from build123d import *

# Parameters (mm, degrees)
SM_BASE_FLANGE_2_DEPTH        = 349
CUT_EXTRUDE_1_DEPTH           = 10
PATTERN_LINEAR_1_COUNT        = 2
PATTERN_LINEAR_1_PITCH        = 251
PATTERN_LINEAR_1_COPY_1_DEPTH = 10


# Sheet-metal steps are written as plain solids
with BuildPart() as part:
    # 草图2 → 基体-法兰2 (new body)
    with BuildSketch(Plane(origin=(0, 0, 0), x_dir=(0, 0, -1), z_dir=(1, 0, 0))):
        Polygon((0, 0), (0, 45.845517328), (4.75, 54.072758664), (5.702627944, 53.522758664), (1.1, 45.550773216), (1.1, 0.294744112), (5.702627944, -7.677241336), (4.75, -8.227241336), align=None)
    extrude(amount=-SM_BASE_FLANGE_2_DEPTH)

    # 草图11 → 切除-拉伸1 (cut)
    with BuildSketch(Plane.XY):
        with BuildLine():
            Line((-46, 14.922758664), (-46, 10.922758664))
            ThreePointArc((-46, 10.922758664), (-49, 7.922758664), (-52, 10.922758664))
            Line((-52, 10.922758664), (-52, 14.922758664))
            ThreePointArc((-52, 14.922758664), (-49, 17.922758664), (-46, 14.922758664))
        make_face()
    cut_extrude_1 = extrude(amount=-CUT_EXTRUDE_1_DEPTH, mode=Mode.SUBTRACT)

    # 镜向1: 切除-拉伸1 across plane
    add(cut_extrude_1.mirror(Plane.ZX.offset(22.922758664)), mode=Mode.SUBTRACT)

    # 阵列(线性)1: 切除-拉伸1 ×2
    with Locations(*[(-i * PATTERN_LINEAR_1_PITCH, 0, 0) for i in range(1, PATTERN_LINEAR_1_COUNT)]):
        add(cut_extrude_1, mode=Mode.SUBTRACT)

    # 阵列(线性)1 copy 1 sketch → 阵列(线性)1 copy 1 (cut)
    with BuildSketch(Plane(origin=(-251, 45.845517328, 0), x_dir=(1, 0, 0), z_dir=(0, 0, 1))):
        with BuildLine():
            Line((-46, -14.922758664), (-46, -10.922758664))
            ThreePointArc((-46, -10.922758664), (-49, -7.922758664), (-52, -10.922758664))
            Line((-52, -10.922758664), (-52, -14.922758664))
            ThreePointArc((-52, -14.922758664), (-49, -17.922758664), (-46, -14.922758664))
        make_face()
    extrude(amount=-PATTERN_LINEAR_1_COPY_1_DEPTH, mode=Mode.SUBTRACT)


solid = part.part
Design review of the part built by this model. Coordinates are the model's own, in mm. A direction names the side the tool comes from. Coordinates: 2 decimals unless noted, no trailing zeros. Loops run counter-clockwise (first coordinate to the right, second up) from the corner with the lowest first, then second, coordinate; pieces in that order, holes last.
Item 1: Clearance check with flat-ended pins moving along their axes: pin 1 (5 mm diameter, centred on x = -159, y = 1, fed in from -Z); pin 2 (5 mm diameter, centred on x = -46, y = 23, fed in from -Z). State where each tip first meets the part, or that it passes through.
Completed:
pin 1: stops at z = -2.14
pin 2: stops at z = -1.1
Item 2: Add section B-B (z = -3.55). Write out the cut boundary in (x, y), and give its area (3 significant figures).
Completed:
outline: (-349, -6.15) - (0, -6.15) - (0, -3.95) - (-349, -3.95) - close; (-349, 49.79) - (0, 49.79) - (0, 51.99) - (-349, 51.99) - close
area: 1,540 mm2
Item 3: Add section D-D (y = 22). Write out the cut boundary in (x, z), and give its area (3 significant figures).
Completed:
outline: (-349, -1.1) - (0, -1.1) - (0, 0) - (-349, 0) - close
area: 384 mm2
Item 4: Wall thickness on L1, parallel to X at y = 13.5, z = -0.55; L2, parallel to Z at x = -34, y = 2; L3, parallel to Y at x = -113, z = -1.9: over which ranges is each line inside the solid? List them lowest first.
Completed:
L1: x = -349 to -303, -297 to -52, -46 to 0
L2: z = -1.1 to 0
L3: y = -3.29 to -1.09, 46.94 to 49.14
Item 5: Draft analysis for pull direction Y (two halves, no side actions). For faces 3 (the flat face through (-172.06, -3.64, -3.37)), 4 (the flat face through (-172, 23, -1.1)), 5 (the flat face through (0, 20.8, -0.5)), 6 (the flat face through (-172.06, 49.9, -2.34)), state which applies: pulls with the +Y half, pulls with the -Y half, needs draft (parallel to the pull), parting line crosses it, or undercut.
Completed:
face 3: undercut
face 4: undercut
face 5: needs draft
face 6: pulls with the +Y half
Item 6: Add section A-A (x = -300). Write out the cut boundary in (y, z), and give its area (3 significant figures).
Completed:
outline: (-8.23, -4.75) - (-7.68, -5.7) - (0.29, -1.1) - (7.92, -1.1) - (7.92, 0) - (0, 0) - close; (17.92, -1.1) - (27.92, -1.1) - (27.92, 0) - (17.92, 0) - close; (37.92, -1.1) - (45.55, -1.1) - (53.52, -5.7) - (54.07, -4.75) - (45.85, 0) - (37.92, 0) - close
area: 48.7 mm2
Item 7: Add section C-C (x = -144.5). Write out the cut boundary in (y, z), and give its area (3 significant figures).
Completed:
outline: (-8.23, -4.75) - (-7.68, -5.7) - (0.29, -1.1) - (45.55, -1.1) - (53.52, -5.7) - (54.07, -4.75) - (45.85, 0) - (0, 0) - close
area: 70.7 mm2
Item 8: For faces 1 (the flat face through (-172.057, -4.171, -2.408)), 2 (the flat face through (-172.06, 49.59, -3.43)), list the 3-axis set-ups (+Z, -Z, +X, -X, +Y, -Y) from which the entire face can be reached by the end or side of a thin tool; tool diameter is ignored.
Completed:
face 1: +Z, +X, -X, -Y
face 2: -Z, +X, -X
